Build history of the part. All positions in model axes, mm. Give positions to 0.01 mm unless a question says otherwise; leave off trailing zeros. Loops run counter-clockwise (first coordinate to the right, second up) from the corner with the lowest first, then second, coordinate; pieces in that order, holes last. Notation, with made-up numbers: M 9,-8.5 L 35,-8.5 A7 cw 35,-1.5 Z; hole C -15,0.5 d10. An arc over 180 degrees is marked long. Put each result on its own line as item: value.
```python
from build123d import *

# Parameters (mm, degrees)
F0_R     = 31.75
F1_DEPTH = 152.4
F2_R     = 25.4
F3_DEPTH = 304.8
F4_R     = 6.35
F5_DEPTH = 31.75


with BuildPart() as f1:
    # F0 (on Top) → F1 (new body, symmetric)
    with BuildSketch(Plane.XY):
        Circle(F0_R)
    extrude(amount=F1_DEPTH, both=True)

    # F2 (on face) → F3 (cut)
    with BuildSketch(Plane(origin=(0, 0, -152.4), x_dir=(1, 0, 0), z_dir=(0, 0, -1))):
        Circle(F2_R)
    extrude(amount=-F3_DEPTH, mode=Mode.SUBTRACT)

    # F4 (on Front) → F5 (cut, symmetric)
    with BuildSketch(Plane.XZ):
        with Locations((0, 82.55)):
            Circle(F4_R)
        with Locations((0, -82.55)):
            Circle(F4_R)
    extrude(amount=F5_DEPTH, both=True, mode=Mode.SUBTRACT)


solid = f1.part
```
Q1. Drop flat-ended pins along their axis: pin 1 Ø5 at (y, z) = (-3.5, -16) entering from +X; pin 2 Ø10 at (x, z) = (0, -82.55) entering from -Y; pin 3 Ø1.5 at (x, z) = (11, -35) entering from -Y; pin 4 Ø8 at (y, z) = (-19.5, 0.5) entering from -X. Give the stop position or say it passes through.
Here are the results:
pin 1: x = 31.73
pin 2: through
pin 3: y = -30.05
pin 4: x = -27.71
Q2. Slice it at C-C (x = -13). List the corners of the cut face in (y, z).
Here are the results:
outline: M -28.97,-152.4 L -21.82,-152.4 L -21.82,152.4 L -28.97,152.4 Z; M 21.82,-152.4 L 28.97,-152.4 L 28.97,152.4 L 21.82,152.4 Z
Q3. Mould opens along X. For faces 1 (the cylindrical face through (-6.883, -30.995, 2.134)), 2 (the cylindrical face through (-5.506, 24.796, -2.134)), 3 (the flat face through (-14.3, 21.3, 152.4)) say: pulls with the +X half, pulls with the -X half, needs draft (parallel to the pull), parting line crosses it, or undercut.
Here are the results:
face 1: parting line crosses it
face 2: undercut
face 3: needs draft
Q4. Probe line 1 (X direction, y = 1, z = -43.5); line 2 (Z direction, x = 0, y = -29); line 3 (Y direction, x = 0, z = -24.5). List the from-to ranges inside material, lowest first. Write a range as from..to.
Here are the results:
line 1: -31.73..-25.38, 25.38..31.73
line 2: -152.4..-88.9, -76.2..76.2, 88.9..152.4
line 3: -31.75..-25.4, 25.4..31.75
Q5. Slice it at D-D (z = 41). List the corners of the cut face in (x, y).
Here are the results:
outline: C 0,0 d63.5; hole C 0,0 d50.8
Q6. Slice it at A-A (y = -4). List the corners of the cut face in (x, z).
Here are the results:
outline: M -31.5,-152.4 L -25.08,-152.4 L -25.08,152.4 L -31.5,152.4 Z; M 25.08,-152.4 L 31.5,-152.4 L 31.5,152.4 L 25.08,152.4 Z
Q7. Slice it at B-B (x = 0). List the corners of the cut face in (y, z), and give its area (3 significant figures).
Here are the results:
outline: M -31.75,-152.4 L -25.4,-152.4 L -25.4,-88.9 L -31.75,-88.9 Z; M -31.75,-76.2 L -25.4,-76.2 L -25.4,76.2 L -31.75,76.2 Z; M -31.75,88.9 L -25.4,88.9 L -25.4,152.4 L -31.75,152.4 Z; M 25.4,-152.4 L 31.75,-152.4 L 31.75,-88.9 L 25.4,-88.9 Z; M 25.4,-76.2 L 31.75,-76.2 L 31.75,76.2 L 25.4,76.2 Z; M 25.4,88.9 L 31.75,88.9 L 31.75,152.4 L 25.4,152.4 Z
area: 3,550 mm²
